Model file for the job. Use its own axes, mm. Face numbers are marked on the shaded views. A direction names the side the tool comes from. Round coordinates to 2 decimals unless told otherwise and drop trailing zeros. Loops run counter-clockwise (first coordinate to the right, second up) from the corner with the lowest first, then second, coordinate; pieces in that order, holes last. Notation, with made-up numbers: (-33.75, 60.5) -> (-25.75, 60.5) arc R17 cw to (-25.75, 76.5) -> close; hole circle Ø6 at (7, 19.5). An arc over 180 degrees is marked (long way). Use a Markdown table: item, result. Add a question column.
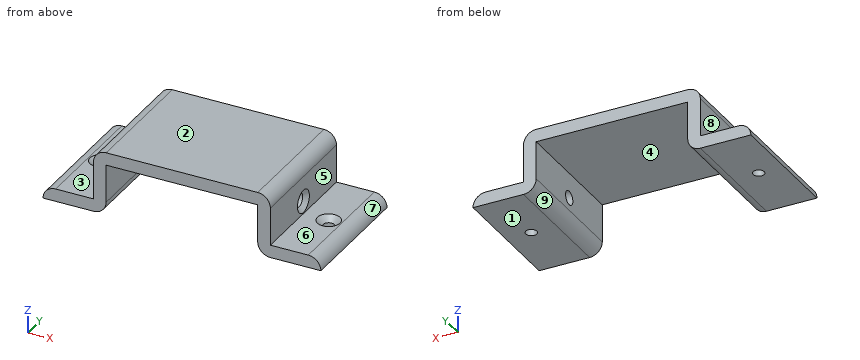
```python
from build123d import *

# Parameters (mm, degrees)
F1_DEPTH             = 50
F4_D                 = 4.4
F4_CSINK_D           = 8.96
F4_CSINK_ANGLE       = 90
F4_ON_F3_D           = 4.4
F4_ON_F3_CSINK_D     = 8.96
F4_ON_F3_CSINK_ANGLE = 90
F6_D                 = 5.5
F6_DEPTH             = 5
F6_CSINK_D           = 9
F6_CSINK_ANGLE       = 90
F6_TIP               = 1.6523667023
F8_D                 = 5.5
F8_DEPTH             = 5
F8_CSINK_D           = 9
F8_CSINK_ANGLE       = 90
F8_TIP               = 1.6523667023
F9_R                 = 4.99999


# Not quite as in the source:
# - a fillet or chamfer is up to 0.001 mm smaller than in the source, because OpenCascade refuses the exact size


with BuildPart() as f1:
    # F0 (on Front) → F1 (new body)
    with BuildSketch(Plane.XZ):
        Polygon((-55, 5), (-55, 0), (-30, 0), (-30, 20), (30, 20), (30, 0), (55, 0), (55, 5), (35, 5), (35, 25), (-35, 25), (-35, 5), align=None)
    extrude(amount=F1_DEPTH)

    # F4 (through all)
    with Locations(Plane.XY.offset(5)):
        with Locations((-45, -25)):
            CounterSinkHole(F4_D / 2, F4_CSINK_D / 2, counter_sink_angle=F4_CSINK_ANGLE)

    # F4 on F3 (through all)
    with Locations(Plane.XY.offset(5)):
        with Locations((45, -25)):
            CounterSinkHole(F4_ON_F3_D / 2, F4_ON_F3_CSINK_D / 2, counter_sink_angle=F4_ON_F3_CSINK_ANGLE)

    # F6
    with Locations(Plane(origin=(-35, 0, 0), x_dir=(0, -1, 0), z_dir=(-1, 0, 0))):
        with Locations((25, 10)):
            CounterSinkHole(F6_D / 2, F6_CSINK_D / 2, depth=F6_DEPTH, counter_sink_angle=F6_CSINK_ANGLE)
            with Locations((0, 0, -(F6_DEPTH + F6_TIP / 2))):  # 118° drill point
                Cone(0, F6_D / 2, F6_TIP, mode=Mode.SUBTRACT)

    # F8
    with Locations(Plane.YZ.offset(35)):
        with Locations((-25, 10)):
            CounterSinkHole(F8_D / 2, F8_CSINK_D / 2, depth=F8_DEPTH, counter_sink_angle=F8_CSINK_ANGLE)
            with Locations((0, 0, -(F8_DEPTH + F8_TIP / 2))):  # 118° drill point
                Cone(0, F8_D / 2, F8_TIP, mode=Mode.SUBTRACT)

    # F9 (radius 5 in the source; OpenCascade refuses exactly that, so slightly less here)
    f9_edges = [f1.edges().sort_by_distance(p)[0] for p in [
        (-30, -25, 0),
        (30, -25, 0),
        (-55, -25, 5),
        (55, -25, 5),
        (-35, -25, 25),
        (35, -25, 25),
    ]]
    fillet(f9_edges, radius=F9_R)


solid = f1.part
```
1) Wall check: probe 1 along Y at (x, z) = (45, 1.9); probe 2 along X at (y, z) = (-5, 19.5); probe 3 along X at (y, z) = (-25, 1.55). Give the ranges that are in metal, low to high. Write a range as from..to.
2) Cut at D-D on z = 4. Write the cut outline in (x, y), and give its area (3 significant figures).
3) Cut at B-B on z = 10. Write the cut outline in (x, y), and give its area (3 significant figures).
4) Tool access for the marked faces 1, 2, 3, 4 and 5: list every direction of +Z, -Z, +X, -X, +Y, -Y with a clear straight run to the whole face (end or side of a thin tool).
5) Pull direction X, two halves, no side cores. Call the marked faces 6, 7, 8 and 9: +X half, -X half, draft (parallel to the pull), parting line (faces both ways), or undercut.
6) Cut at A-A on x = -45. Write the cut outline in (y, z), and give its area (3 significant figures).
7) Pin check, flat tips, straight feed: pin 1 Ø1.5 at (y, z) = (-44.5, 16.5) entering from +X; pin 2 Ø5 at (x, y) = (28, -39.5) entering from -Z; pin 3 Ø3.5 at (x, y) = (45, -25) entering from -Z; pin 4 Ø7 at (y, z) = (-25, 10) entering from -X. Stop position of each tip, or through.
Established:
| question | item | result |
|---|---|---|
| 1 | probe 1 | y = -50..-27.2, -22.8..0 |
| 1 | probe 2 | x = -35..-30, 30..35 |
| 1 | probe 3 | x = -54.75..-47.2, -42.8..-31.38, 31.38..42.8, 47.2..54.75 |
| 2 | outline | (-53, -50) -> (-30.1, -50) -> (-30.1, 0) -> (-53, 0) -> close; (30.1, -50) -> (53, -50) -> (53, 0) -> (30.1, 0) -> close; hole circle Ø6.96 at (-45, -25); hole circle Ø6.96 at (45, -25) |
| 2 | area | 2,210 mm^2 |
| 3 | outline | (-35, -50) -> (-30, -50) -> (-30, -27.75) -> (-33.25, -27.75) -> (-35, -29.5) -> close; (-35, -20.5) -> (-33.25, -22.25) -> (-30, -22.25) -> (-30, 0) -> (-35, 0) -> close; (30, -50) -> (35, -50) -> (35, -29.5) -> (33.25, -27.75) -> (30, -27.75) -> close; (30, -22.25) -> (33.25, -22.25) -> (35, -20.5) -> (35, 0) -> (30, 0) -> close |
| 3 | area | 439 mm^2 |
| 4 | face 1 | -Z, +X, -X, +Y, -Y |
| 4 | face 2 | +Z, +X, -X, +Y, -Y |
| 4 | face 3 | +Z, -X, +Y, -Y |
| 4 | face 4 | -Z, +Y, -Y |
| 4 | face 5 | +Z, +X, +Y, -Y |
| 5 | face 6 | draft |
| 5 | face 7 | +X half |
| 5 | face 8 | -X half |
| 5 | face 9 | undercut |
| 6 | outline | (-50, 0) -> (-27.2, 0) -> (-27.2, 2.72) -> (-29.48, 5) -> (-50, 5) -> close; (-22.8, 0) -> (0, 0) -> (0, 5) -> (-20.52, 5) -> (-22.8, 2.72) -> close |
| 6 | area | 223 mm^2 |
| 7 | pin 1 | stops at x = 35 |
| 7 | pin 2 | stops at z = 2.82 |
| 7 | pin 3 | passes through |
| 7 | pin 4 | stops at x = -34 |
